Autodesk Inventor part; units mm, degrees
ref_plane "YZ Plane" through (0, 0, 0) normal (1, 0, 0) x (0, 1, 0)
ref_plane "XZ Plane" through (0, 0, 0) normal (0, 1, 0) x (-1, 0, 0)
ref_plane "XY Plane" through (0, 0, 0) normal (0, 0, 1) x (1, 0, 0)
sketch "Sketch1" plane through (0, 0, 0) normal (0, 1, 0) x (-1, 0, 0)
  line L0 (100, -16.077) -> (100, -30)
  line L1 (0, -5) -> (0, 0)
  line L2 (0, 0) -> (40, 0)
  line L3 (40, 0) -> (100, -16.077)
  line L4 (100, -16.077) -> (100, -26.077)
  line L5 (45, -30) -> (55, -30)
  arc A0 (45, -30) -> (34.4399, -15.6721) centre (30, -30) ccw
  line L6 (0, -5) -> (34.4399, -15.6721)
  arc A1 (85.7288, -30) -> (59.2712, -30) centre (72.5, -45) ccw
  line L7 (100, -30) -> (85.7288, -30)
  line L8 (59.2712, -30) -> (45, -30)
extrude "Extrusion1" add sketch "Sketch1" along normal blind 15
sketch "Sketch2" plane through (0, 15, 0) normal (0, 1, 0) x (1, 0, 0)
  line L0 (0, 0) -> (0, 5)
  circle A0 centre (-5, 2.5) radius 1.5
  circle A1 centre (-35, 10) radius 1.5
  dimension "d14" = 3
  dimension "d17" = 3
extrude "Extrusion2" cut sketch "Sketch2" against normal blind 15
sketch "Sketch3" plane through (-40, 0, 0) normal (0, 0, 1) x (1, 0, 0)
  line L0 (40, 0) -> (40, 15)
  line L1 (40, 5) -> (0, 5)
  line L2 (0, 5) -> (0, 10)
  line L3 (0, 10) -> (40, 10)
  line L4 (40, 10) -> (40, 5)
  dimension "d20" = 5
  dimension "d21" = 40
  dimension "d22" = 5
extrude "Extrusion3" cut sketch "Sketch3" against normal blind 44.75
properties part number "gripper3"
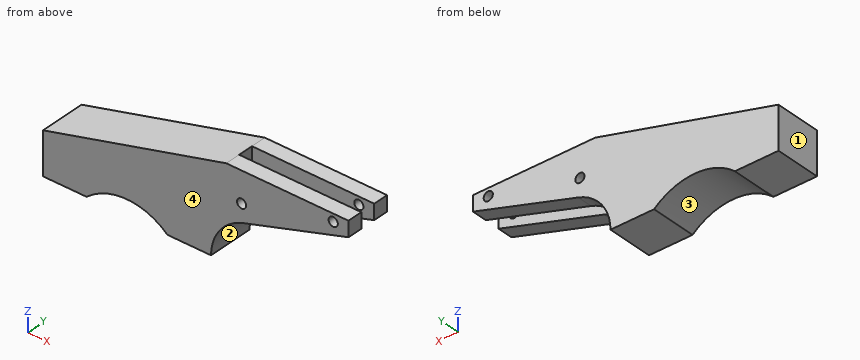
Check sheet for the modelled part. Datum: model origin and axes. Units: mm. Face numbers are marked on the shaded views. Round coordinates to 2 decimals unless told otherwise and drop trailing zeros. Loops run counter-clockwise (first coordinate to the right, second up) from the corner with the lowest first, then second, coordinate; pieces in that order, holes last.
1. Sectioned sample at A-A on y = 12.5. Record the boundary of the cut face in (x, z), and give its area (3 significant figures).
2. Sectioned sample at C-C on z = -10. Record the boundary of the cut face in (x, y), and give its area (3 significant figures).
3. Mould release check, pull along X, two halves, no side actions. Record for the marked faces 1, 2, 3 and 4: released by +X, released by -X, zero draft, split by the parting line, or undercut.
4. Gauge pin test, flat ends, axial feed: pin 1 Ø3 at (x, z) = (-29.5, -17) entering from -Y; pin 2 Ø1 at (y, z) = (3, -25) entering from +X; pin 3 Ø1 at (x, y) = (-72.5, 10.5) entering from +Z; pin 4 Ø2.5 at (y, z) = (8.5, -6.5) entering from +X. Record the tip position at first contact, or that the pin passes through.
5. Sectioned sample at D-D on y = 6. Record the boundary of the cut face in (x, z).
6. Scan lines: probe 1 along Y at (x, z) = (-36, -14); probe 2 along Z at (x, y) = (-5, 13.55); probe 3 along Z at (x, y) = (-35, 11.65). Record each from-to range of solid material in increasing order.
7. Sectioned sample at B-B on x = -5. Record the boundary of the cut face in (y, z).
Recorded:
1. outline: (-100, -30) - (-85.73, -30) arc R20 cw to (-59.27, -30) - (-45, -30) arc R15 cw to (-34.44, -15.67) - (0, -5) - (0, 0) - (-40, 0) - (-100, -16.08) - close; hole circle Ø3 at (-35, -10); hole circle Ø3 at (-5, -2.5)
1. area: 1,620 mm2
2. outline: (-77.32, 0) - (-36.5, 0) - (-36.5, 5) - (-40, 5) - (-40, 10) - (-36.5, 10) - (-36.5, 15) - (-77.32, 15) - close; (-33.5, 0) - (-16.14, 0) - (-16.14, 5) - (-33.5, 5) - close; (-33.5, 10) - (-16.14, 10) - (-16.14, 15) - (-33.5, 15) - close
2. area: 768 mm2
3. face 1: released by -X
3. face 2: released by +X
3. face 3: undercut
3. face 4: zero draft
4. pin 1: passes through
4. pin 2: stops at x = -43.96
4. pin 3: stops at z = -8.57
4. pin 4: stops at x = -40
5. outline: (-100, -30) - (-85.73, -30) arc R20 cw to (-59.27, -30) - (-45, -30) arc R15 cw to (-40, -18.82) - (-40, 0) - (-100, -16.08) - close
6. probe 1: y = 0 to 5, 10 to 15
6. probe 2: z = -6.55 to -4, -1 to 0
6. probe 3: z = -15.86 to -11.5, -8.5 to 0
7. outline: (0, -6.55) - (5, -6.55) - (5, -4) - (0, -4) - close; (0, -1) - (5, -1) - (5, 0) - (0, 0) - close; (10, -6.55) - (15, -6.55) - (15, -4) - (10, -4) - close; (10, -1) - (15, -1) - (15, 0) - (10, 0) - close
